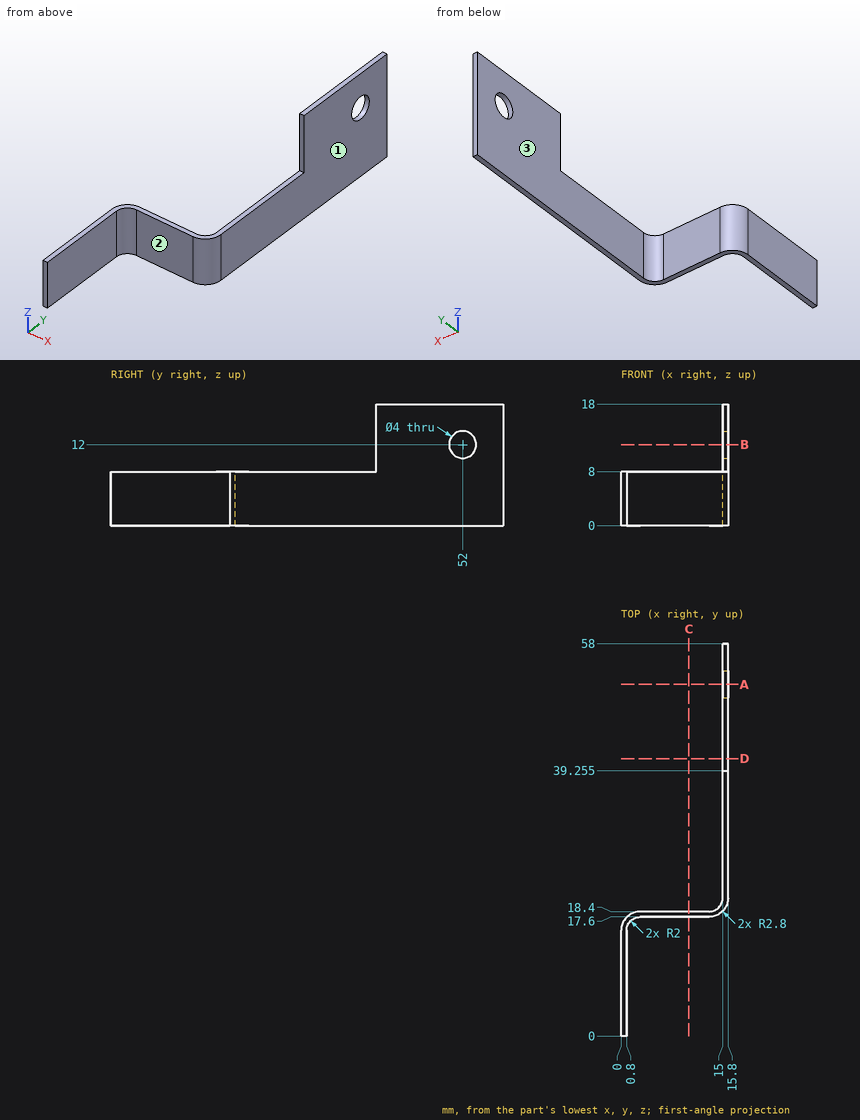
The drawing under review shows one solid part. Ordinate dimensions are in mm from its lowest x, y, z. A direction names the side the tool comes from. Coordinates: 2 decimals unless noted, no trailing zeros. Order: outer loops, then holes, each group sorted by start corner. A loop starts at its lowest first (then second) coordinate and runs counter-clockwise, first axis right, second up. Notation, with made-up numbers: (54.25, 39) -> (101.25, 39) arc R24 ccw to (101.25, 50) -> close; hole circle Ø3 at (53, 63.25). An arc over 180 degrees is marked (long way). Answer in a Markdown table with one row per item.
(1) Machinability: for the marked faces 1, 2 and 3, which of the approach directions +Z, -Z, +X, -X, +Y, -Y give a long, thin tool a straight path to every point of the face, cutting with its end or side? Answer none if there is none.
Answers:
| item | result |
|---|---|
| face 1 | +Z, -Z, +X, +Y, -Y |
| face 2 | +Z, -Z, +X, -Y |
| face 3 | +Z, -Z, -X, +Y |
(2) Consider section B-B (z = 12). Write out the cut boundary in (x, y) (1 decimal).
Answers:
| item | result |
|---|---|
| outline | (15, 39.3) -> (15.8, 39.3) -> (15.8, 50) -> (15, 50) -> close; (15, 54) -> (15.8, 54) -> (15.8, 58) -> (15, 58) -> close |
(3) Consider section C-C (x = 10). Write out the cut boundary in (y, z).
Answers:
| item | result |
|---|---|
| outline | (17.6, 0) -> (18.4, 0) -> (18.4, 8) -> (17.6, 8) -> close |
(4) Insertion check: pin 1 (10 mm diameter, centred on y = 15.5, z = 15.5, fed in from -X); pin 2 (9 mm diameter, centred on x = 9.5, z = 4.5, fed in from -Y); pin 3 (9 mm diameter, centred on x = 7, z = 5, fed in from +Y); pin 4 (6.5 mm diameter, centred on y = 5.5, z = 5, fed in from +X). Each pin has a flat end and moves straight along its axis. Give the tip position at first contact, or say it passes through.
Answers:
| item | result |
|---|---|
| pin 1 | through |
| pin 2 | y = 17.6 |
| pin 3 | y = 18.4 |
| pin 4 | x = 0.8 |
(5) Wall thickness on line 1 along X through (y, z) = (12, 6.5); line 2 along X through (y, z) = (44, 16); line 3 along Y through (x, z) = (15.65, 12) (1 decimal): over which ranges is each line inside the solid? List them lowest first.
Answers:
| item | result |
|---|---|
| line 1 | 0 to 0.8 |
| line 2 | 15 to 15.8 |
| line 3 | 39.3 to 50, 54 to 58 |
(6) Consider section A-A (y = 52). Write out the cut boundary in (x, z), plus the area to 3 significant figures.
Answers:
| item | result |
|---|---|
| outline | (15, 0) -> (15.8, 0) -> (15.8, 10) -> (15, 10) -> close; (15, 14) -> (15.8, 14) -> (15.8, 18) -> (15, 18) -> close |
| area | 11.2 mm² |
(7) Consider section D-D (y = 41). Write out the cut boundary in (x, z).
Answers:
| item | result |
|---|---|
| outline | (15, 0) -> (15.8, 0) -> (15.8, 18) -> (15, 18) -> close |
